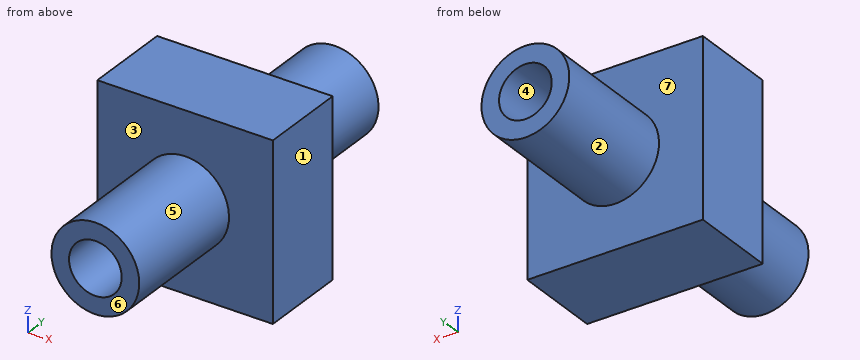
```python
from build123d import *

# Parameters (mm, degrees)
F0_W     = 100
F0_H     = 100
F1_DEPTH = 50
F2_W     = 200
F2_H     = 25
F5_D     = 30


with BuildPart() as f1:
    # F0 (on Front) → F1 (new body)
    with BuildSketch(Plane.XZ):
        Rectangle(F0_W, F0_H)
    extrude(amount=-F1_DEPTH)

    # F2 (on Right) → F3 (revolve)
    with BuildSketch(Plane.YZ):
        with Locations((25, 12.5)):
            Rectangle(F2_W, F2_H)
    revolve(axis=Axis((0, 49.7826111294, 0), (0, 1, 0)))

    # F5 (through all)
    with Locations(Plane.XZ.offset(75)):
        with Locations((0, 0)):
            Hole(F5_D / 2)


solid = f1.part
```
Could you check a few things on this model? Use its own coordinates, in mm. Face numbers are marked on the shaded views. A direction names the side the tool comes from. Give positions to 0.01 mm unless a question says otherwise; leave off trailing zeros. Order: outer loops, then holes, each group sorted by start corner. A loop starts at its lowest first (then second) coordinate and runs counter-clockwise, first axis right, second up.
Q1. Suppose I cut it at C-C, the plane y = 19. Write out the boundary of the cut face in (x, z).
Q2. We'd pull the mould along X, two halves only. Please class the marked faces 1, 2, 3 and 4: +X half, -X half, draft (parallel to the pull), parting line (faces both ways), or undercut.
Q3. Suppose I cut it at B-B, the plane x = 0. Write out the boundary of the cut face in (y, z).
Q4. I'm going to push flat-ended pins straight in: P1, Ø1.5, axis at x = 17.5, y = 73.5, coming from the +Z side; P2, Ø6, axis at y = 89, z = -15.5, coming from the -X side; P3, Ø1.5, axis at x = 19, z = -16.5, coming from the -Y side; P4, Ø2, axis at x = 11, y = 58, coming from the -Z side. Where does each tip first touch, or does it pass through?
Q5. Suppose I cut it at D-D, the plane x = -33.5. Write out the boundary of the cut face in (y, z), and give its area (3 significant figures).
Q6. If I drill on line 1 along Z through (x, y) = (0, 34); line 2 along X through (y, z) = (70.5, -0.5) (3 decimals); line 3 along Y through (x, z) = (26.5, -23.5), over which ranges is the centre line in solid material (lowest first)?
Q7. Suppose I cut it at A-A, the plane z = 0. Write out the boundary of the cut face in (x, y).
Q8. For the marked faces 5, 6 and 7, which set-ups out of +Z, -Z, +X, -X, +Y, -Y let a thin tool reach every point of the face, with its end or its side?
Solution:
1. outline: (-50, -50) - (50, -50) - (50, 50) - (-50, 50) - close; hole circle Ø30 at (0, 0)
2. face 1: +X half
2. face 2: parting line
2. face 3: draft
2. face 4: undercut
3. outline: (-75, -25) - (0, -25) - (0, -50) - (50, -50) - (50, -25) - (125, -25) - (125, -15) - (-75, -15) - close; (-75, 15) - (125, 15) - (125, 25) - (50, 25) - (50, 50) - (0, 50) - (0, 25) - (-75, 25) - close
4. P1: stops at z = 18.56
4. P2: stops at x = -21.65
4. P3: stops at y = -75
4. P4: stops at z = -22.91
5. outline: (0, -50) - (50, -50) - (50, 50) - (0, 50) - close
5. area: 5,000 mm2
6. line 1: z = -50 to -15, 15 to 50
6. line 2: x = -24.995 to -14.992, 14.992 to 24.995
6. line 3: y = 0 to 50
7. outline: (-50, 0) - (-25, 0) - (-25, -75) - (-15, -75) - (-15, 125) - (-25, 125) - (-25, 50) - (-50, 50) - close; (15, -75) - (25, -75) - (25, 0) - (50, 0) - (50, 50) - (25, 50) - (25, 125) - (15, 125) - close
8. face 5: -Y
8. face 6: +Z, -Z, +X, -X, -Y
8. face 7: +Y
